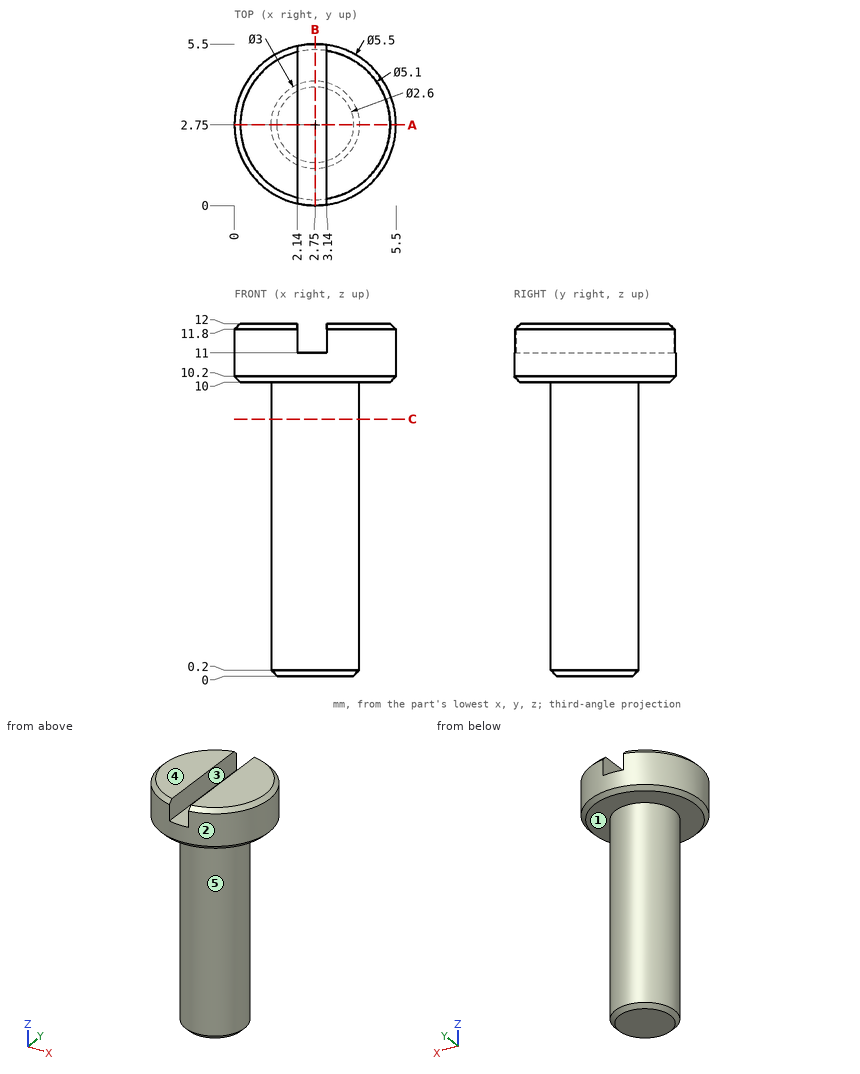
Input: dimensioned drawing with shaded views. Units: mm. Origin: part minimum x, y, z. A direction names the side the tool comes from. Give positions to 0.01 mm unless a question says otherwise; leave off trailing zeros. Write each loop counter-clockwise with the first axis right and the second up, starting at its lowest first coordinate (ties: lowest second). Pieces come first, ordered by that corner, then holes. Notation, with made-up numbers: (20.25, -26.75) -> (70.25, -26.75) arc R25 cw to (70.25, -4.75) -> close; hole circle Ø7 at (14.25, 24). An arc over 180 degrees is marked (long way). Answer as a JSON object with one key per item and string values.
1. Ray query, probe 1 along Z at (x, y) = (2.2, 0.9); probe 2 along Z at (x, y) = (1.75, 5); probe 3 along X at (y, z) = (2, 4.25). Return the intervals inside material, ascending. Write a range as from..to.
Ans:
{"probe 1": "z = 10..11", "probe 2": "z = 10..12", "probe 3": "x = 1.45..4.05"}
2. Contact query for flat-ended pins moving along their axis: pin 1 (1.1 mm diameter, centred on y = 1.5, z = 11.5, fed in from +X); pin 2 (1 mm diameter, centred on y = 1, z = 8.5, fed in from +X); pin 3 (1 mm diameter, centred on y = 2, z = 10, fed in from -X). Output: stop coordinate, or through.
Ans:
{"pin 1": "stops at x = 5.41", "pin 2": "stops at x = 3.58", "pin 3": "stops at x = 0.02"}
3. Access query for the marked faces 4 and 5. Directions: +Z, -Z, +X, -X, +Y, -Y. A direction counts if a zero-diameter tool reaches every point of the face in a straight line with its end or side. Return the directions, or none.
Ans:
{"face 4": "+Z, +X, -X, +Y, -Y", "face 5": "-Z"}
4. Cut plane A-A on y = 2.75. Output: boundary loops of the cut face in (x, z), and give its area (3 significant figures).
Ans:
{"outline": "(0, 10.2) -> (0.2, 10) -> (1.25, 10) -> (1.25, 0.2) -> (1.45, 0) -> (4.05, 0) -> (4.25, 0.2) -> (4.25, 10) -> (5.3, 10) -> (5.5, 10.2) -> (5.5, 11.8) -> (5.3, 12) -> (3.14, 12) -> (3.14, 11) -> (2.14, 11) -> (2.14, 12) -> (0.2, 12) -> (0, 11.8) -> close", "area": "39.9 mm^2"}
5. Cut plane B-B on x = 2.75. Output: boundary loops of the cut face in (y, z).
Ans:
{"outline": "(0, 10.2) -> (0.2, 10) -> (1.25, 10) -> (1.25, 0.2) -> (1.45, 0) -> (4.05, 0) -> (4.25, 0.2) -> (4.25, 10) -> (5.3, 10) -> (5.5, 10.2) -> (5.5, 11) -> (0, 11) -> close"}
6. Cut plane C-C on z = 8.75. Output: boundary loops of the cut face in (x, y).
Ans:
{"outline": "circle Ø3 at (2.75, 2.75)"}
7. Mould query, pull axis X, two halves, no side actions, for the marked faces 1, 2 and 3. Classes: pulls with the +X half, pulls with the -X half, needs draft (parallel to the pull), parting line crosses it, or undercut.
Ans:
{"face 1": "needs draft", "face 2": "parting line crosses it", "face 3": "undercut"}
